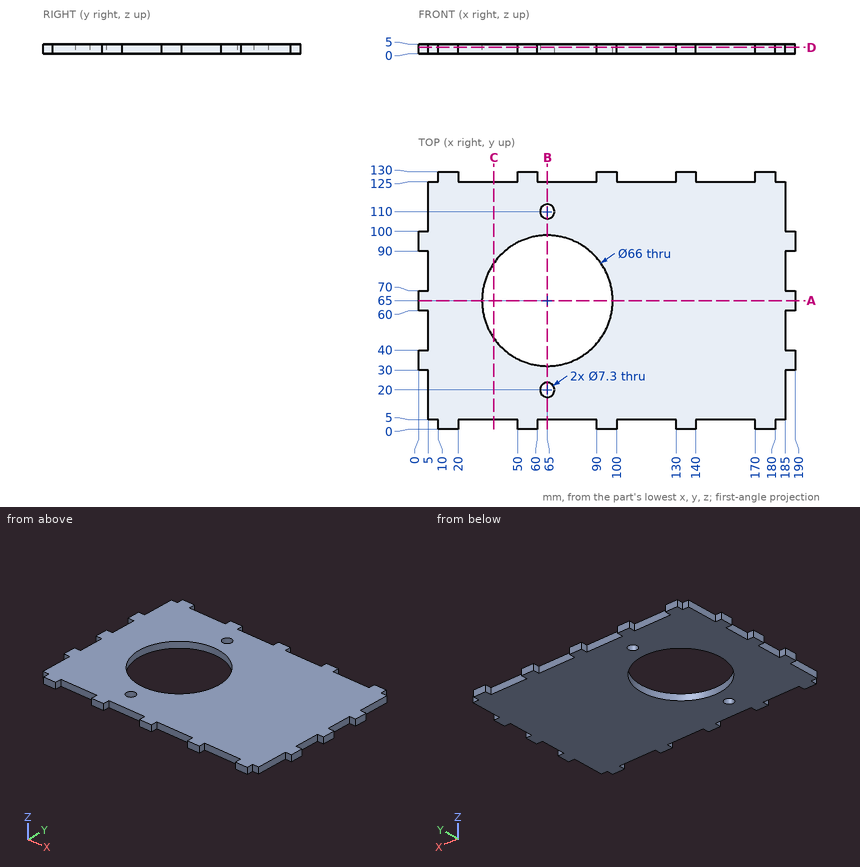
Geometry check sheet. Reference: drawing and pictorial views, mm from the part's lowest x, y, z. Coordinates: 2 decimals unless noted, no trailing zeros. Write each loop counter-clockwise with the first axis right and the second up, starting at its lowest first coordinate (ties: lowest second). Pieces come first, ordered by that corner, then holes. Notation, with made-up numbers: (-30.75, 45) - (4.25, 45) arc R16 cw to (4.25, 70) - close; hole circle Ø11 at (13.25, -22.5). An arc over 180 degrees is marked (long way). Write item = value, one per line.
Q1. Material ranges on L1, parallel to Y at x = 65, z = 2.05; L2, parallel to Y at x = 141, z = 0.7; L3, parallel to Y at x = 38, z = 0.5, recorded low to high. Write a range as from..to.
Answer:
L1 = 5..16.35, 23.65..32, 98..106.35, 113.65..125
L2 = 5..125
L3 = 5..46.03, 83.97..125
Q2. Cross-section at B-B (x = 65). Enter the section's corners in (y, z).
Answer:
outline = (5, 0) - (16.35, 0) - (16.35, 5) - (5, 5) - close; (23.65, 0) - (32, 0) - (32, 5) - (23.65, 5) - close; (98, 0) - (106.35, 0) - (106.35, 5) - (98, 5) - close; (113.65, 0) - (125, 0) - (125, 5) - (113.65, 5) - close
Q3. Cross-section at A-A (y = 65). Enter the section's corners in (x, z).
Answer:
outline = (0, 0) - (32, 0) - (32, 5) - (0, 5) - close; (98, 0) - (190, 0) - (190, 5) - (98, 5) - close
Q4. Cross-section at C-C (x = 38). Enter the section's corners in (y, z).
Answer:
outline = (5, 0) - (46.03, 0) - (46.03, 5) - (5, 5) - close; (83.97, 0) - (125, 0) - (125, 5) - (83.97, 5) - close
Q5. Cross-section at D-D (z = 3.3). Give the number of separate pieces and of enclosed holes in the cut face, plus the area to 3 significant figures.
Answer:
separate_pieces = 1
enclosed_holes = 3
area = 18,900 mm²
Q6. Go/stop test with flat-tipped pins: pin 1 Ø2.5 at (y, z) = (127, 2) entering from +X; pin 2 Ø1.5 at (x, z) = (95.5, 3.5) entering from -Y; pin 3 Ø2.5 at (x, z) = (2.5, 3) entering from +Y; pin 4 Ø2.5 at (y, z) = (114.5, 2.5) entering from +X. Record where each tip stops, or that it passes through.
Answer:
pin_1 = 180
pin_2 = 0
pin_3 = 100
pin_4 = 185
